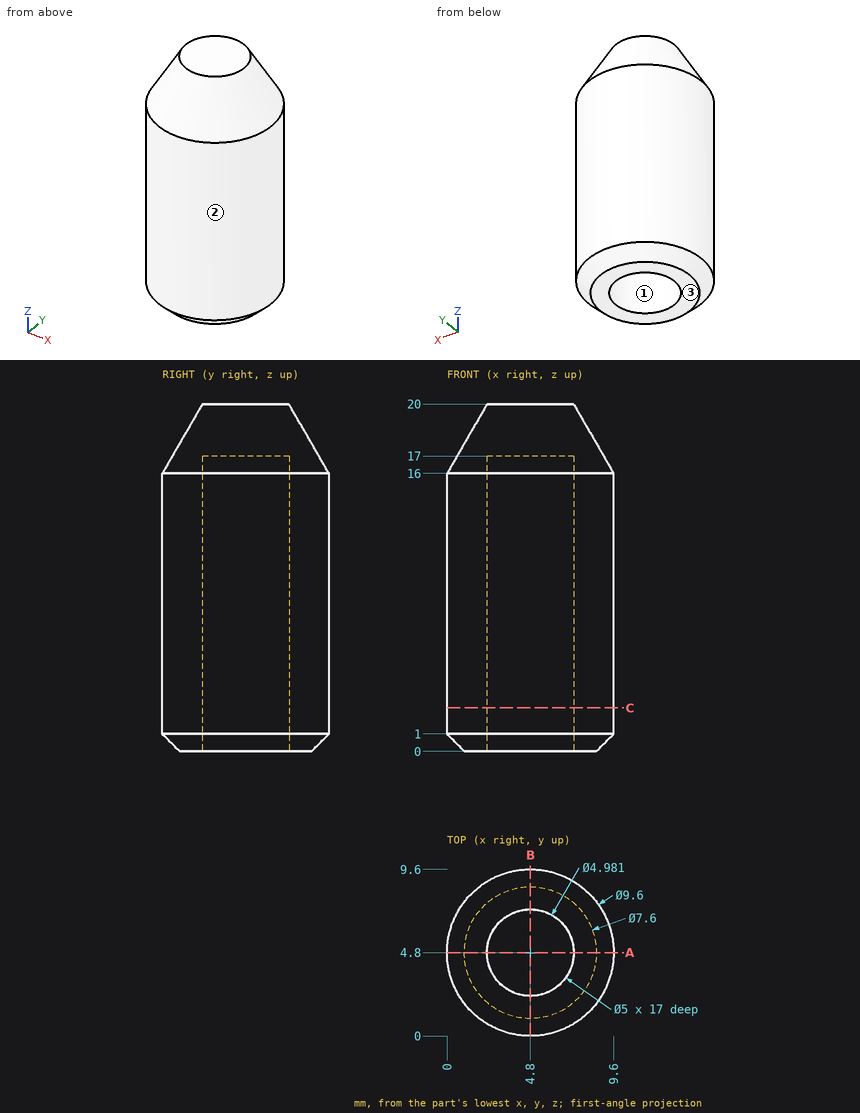
Print and shaded views of the part. All mm, measured from the part's lowest x, y and z. Round coordinates to 2 decimals unless told otherwise and drop trailing zeros. Write each loop counter-clockwise with the first axis right and the second up, starting at its lowest first coordinate (ties: lowest second). Pieces come first, ordered by that corner, then holes.
Item 1: Cut at C-C, the plane z = 2.5. Give the cut face in (x, y).
Results:
outline: circle Ø9.6 at (4.8, 4.8); hole circle Ø5 at (4.8, 4.8)
Item 2: Cut at A-A, the plane y = 4.8. Give the cut face in (x, z).
Results:
outline: (0, 1) - (1, 0) - (2.3, 0) - (2.3, 17) - (7.3, 17) - (7.3, 0) - (8.6, 0) - (9.6, 1) - (9.6, 16) - (7.29, 20) - (2.31, 20) - (0, 16) - close
Item 3: Probe L1, parallel to X at y = 4.8, z = 12.75; L2, parallel to Z at x = 4, y = 6.25; L3, parallel to X at y = 2.5, z = 6.25 (1 decimal). List the from-to ranges inside material, lowest first.
Results:
L1: x = 0 to 2.3, 7.3 to 9.6
L2: z = 17 to 20
L3: x = 0.6 to 3.8, 5.8 to 9
Item 4: Two-plate mould, pull along Y, no slides. Class the marked faces 1, 2 and 3: +Y half, -Y half, draft (parallel to the pull), parting line (faces both ways), or undercut.
Results:
face 1: undercut
face 2: parting line
face 3: draft
Item 5: Drop flat-ended pins along their axis: pin 1 Ø3 at (x, z) = (6.5, 11.5) entering from -Y; pin 2 Ø2 at (x, y) = (2, 3.5) entering from -Z; pin 3 Ø3 at (x, y) = (4.8, 4.8) entering from -Z; pin 4 Ø1 at (x, y) = (2, 8) entering from +Z (1 decimal). Give the stop position or say it passes through.
Results:
pin 1: stops at y = 0
pin 2: stops at z = 0
pin 3: stops at z = 17
pin 4: stops at z = 17.8
